CAD build for the part. Positions are in the model's coordinates, mm. A direction names the side the tool comes from. Round coordinates to 2 decimals unless told otherwise and drop trailing zeros. Order: outer loops, then holes, each group sorted by start corner. A loop starts at its lowest first (then second) coordinate and runs counter-clockwise, first axis right, second up. Notation, with made-up numbers: (34.5, 5) -> (83.5, 5) arc R28 ccw to (83.5, 25) -> close; hole circle Ø4 at (43, 5). An arc over 180 degrees is marked (long way). Return JSON: item names as keys, results as strings. Group by question number.
Q1. Cut at B-B (x = -155.5). Write the cut outline in (y, z).
Q2. Mould opens along Z. For faces 1 (the flat face through (185, 13.5, -14)), 2 (the flat face through (14, 13.5, 185)), 3 (the flat face through (161, 32, 37.5)) say: +Z half, -Z half, draft (parallel to the pull), parting line (faces both ways), or undercut.
Q3. Flat gauge pins, fed straight in: pin 1 (3 mm diameter, centred on x = -183.5, z = -15.5, fed in from +Y); pin 2 (8 mm diameter, centred on y = 81.5, z = -47, fed in from -X); pin 3 (1.5 mm diameter, centred on y = 43.5, z = -18.5, fed in from -X). Where does each tip first touch, or does it go through?
Q4. Which spindle directions (+Z, -Z, +X, -X, +Y, -Y) get a long thin tool onto all of the face, cutting with end or side? Do faces 4 (the flat face through (33, 65, 157)), 5 (the flat face through (-120.878, 44.58, -71.982)), 6 (the flat face through (-172, 10, -1)). Say none if no direction does.
Q5. Cut at A-A (x = 0). Write the cut outline in (y, z).
Q6. Probe line 1 along X through (y, z) = (50.5, 162); line 2 along Y through (x, z) = (-61, 22); line 3 along Z through (x, y) = (71, 27.5). List the from-to ranges inside material, lowest first.
from build123d import *

# Parameters (mm, degrees)
SKETCH1_R                    = 150
BOSS_EXTRUDE1_DEPTH          = 75
CHAMFER1_SIZE                = 10
BOSS_EXTRUDE2_START          = -75
BOSS_EXTRUDE2_DEPTH          = 10
CHAMFER2_SIZE                = 10
BOSS_EXTRUDE3_DEPTH          = 10
BOSS_EXTRUDE4_DEPTH          = 3.5
CIRPATTERN1_COUNT            = 4
CIRPATTERN1_COPY_1_DEPTH     = 10
CIRPATTERN1_COPY_2_DEPTH     = 10
CIRPATTERN1_COPY_3_DEPTH     = 10
CIRPATTERN1_COPY_4_DEPTH     = 3.5
CIRPATTERN1_COPY_5_DEPTH     = 3.5
CIRPATTERN1_COPY_6_DEPTH     = 3.5
CHAMFER2_OF_CIRPATTERN1_SIZE = 10
CUT_EXTRUDE1_START           = -60
CUT_EXTRUDE1_DEPTH           = 60
CIRPATTERN3_COUNT            = 4
SKETCH15_R                   = 110
BOSS_EXTRUDE6_DEPTH          = 9
BOSS_EXTRUDE6_TAPER          = 45
SKETCH16_R                   = 15
BOSS_EXTRUDE7_DEPTH          = 20


# Read off the part's stored shape, not the designer's step: Cut-Extrude1
with BuildPart() as part:
    # Sketch1 → Boss-Extrude1 (new body)
    with BuildSketch(Plane(origin=(0, 0, 0), x_dir=(1, 0, 0), z_dir=(0, 1, 0))):
        with Locations(Location((0, 0, 0), (0, 0, 270))):
            Circle(SKETCH1_R)
    extrude(amount=BOSS_EXTRUDE1_DEPTH)

    # Chamfer1
    chamfer1_edges = [part.edges().sort_by_distance(p)[0] for p in [
        (0, 75, -150),
    ]]
    chamfer(chamfer1_edges, length=CHAMFER1_SIZE)

    # Sketch2 → Boss-Extrude2 (add)
    with BuildSketch(Plane(origin=(0, 75, 0), x_dir=(1, 0, 0), z_dir=(0, 1, 0)).offset(BOSS_EXTRUDE2_START)):
        with BuildLine():
            ThreePointArc((-145.236875483, -37.5), (-148.80445444, -18.900643872), (-150, 0))
            Line((-150, 0), (-195.236875483, 0))
            Line((-195.236875483, 0), (-195.236875483, -37.5))
            Line((-195.236875483, -37.5), (-145.236875483, -37.5))
        make_face()
        with BuildLine():
            Line((-195.236875483, 0), (-150, 0))
            ThreePointArc((-150, 0), (-148.80445444, 18.900643872), (-145.236875483, 37.5))
            Line((-145.236875483, 37.5), (-195.236875483, 37.5))
            Line((-195.236875483, 37.5), (-195.236875483, 0))
        make_face()
    boss_extrude2 = extrude(amount=BOSS_EXTRUDE2_DEPTH)

    # Chamfer2
    chamfer2_edges = [part.edges().sort_by_distance(p)[0] for p in [
        (-195.236875483, 5, -37.5),
        (-195.236875483, 5, 37.5),
    ]]
    chamfer(chamfer2_edges, length=CHAMFER2_SIZE)

    # Sketch5 → Boss-Extrude3 (add)
    with BuildSketch(Plane.XY.offset(37.5)):
        Polygon((-145.236875483, 10), (-145.236875483, 65), (-168.236875483, 65), (-185.236875483, 10), align=None)
    boss_extrude3 = extrude(amount=-BOSS_EXTRUDE3_DEPTH)

    # Sketch7 → Boss-Extrude4 (add)
    with BuildSketch(Plane(origin=(0, 10, 0), x_dir=(1, 0, 0), z_dir=(0, 1, 0))):
        Polygon((-180.034917045, -11.010056312), (-185.225263454, -8), (-190.427221891, -10.989943688), (-190.43883392, -16.989943688), (-185.248487512, -20), (-180.046529075, -17.010056312), align=None)
    boss_extrude4 = extrude(amount=BOSS_EXTRUDE4_DEPTH)

    # Mirror2: Boss-Extrude3, Boss-Extrude4 across plane
    add(boss_extrude3.mirror(Plane.XY))
    add(boss_extrude4.mirror(Plane.XY))

    # CirPattern1: Boss-Extrude2, Boss-Extrude3, Boss-Extrude4 ×4 about axis
    cirpattern1_axis = Axis((0, 0, 0), (0, 1, 0))
    add([boss_extrude2.rotate(cirpattern1_axis, i * 360 / CIRPATTERN1_COUNT) for i in range(1, CIRPATTERN1_COUNT)])
    add([boss_extrude3.rotate(cirpattern1_axis, i * 360 / CIRPATTERN1_COUNT) for i in range(1, CIRPATTERN1_COUNT)])
    add([boss_extrude4.rotate(cirpattern1_axis, i * 360 / CIRPATTERN1_COUNT) for i in range(1, CIRPATTERN1_COUNT)])

    # CirPattern1 copy 1 sketch → CirPattern1 copy 1 (add)
    with BuildSketch(Plane(origin=(-37.5, 0, 0), x_dir=(0, 0, -1), z_dir=(-1, 0, 0))):
        Polygon((-145.236875483, -10), (-145.236875483, -65), (-168.236875483, -65), (-185.236875483, -10), align=None)
    extrude(amount=-CIRPATTERN1_COPY_1_DEPTH)

    # CirPattern1 copy 2 sketch → CirPattern1 copy 2 (add)
    with BuildSketch(Plane(origin=(0, 0, 37.5), x_dir=(-1, 0, 0), z_dir=(0, 0, 1))):
        Polygon((-145.236875483, -10), (-145.236875483, -65), (-168.236875483, -65), (-185.236875483, -10), align=None)
    extrude(amount=-CIRPATTERN1_COPY_2_DEPTH)

    # CirPattern1 copy 3 sketch → CirPattern1 copy 3 (add)
    with BuildSketch(Plane(origin=(37.5, 0, 0), x_dir=(0, 0, 1), z_dir=(1, 0, 0))):
        Polygon((-145.236875483, -10), (-145.236875483, -65), (-168.236875483, -65), (-185.236875483, -10), align=None)
    extrude(amount=-CIRPATTERN1_COPY_3_DEPTH)

    # CirPattern1 copy 4 sketch → CirPattern1 copy 4 (add)
    with BuildSketch(Plane(origin=(0, 10, 0), x_dir=(0, 0, -1), z_dir=(0, 1, 0))):
        Polygon((-180.034917045, 11.010056312), (-185.225263454, 8), (-190.427221891, 10.989943688), (-190.43883392, 16.989943688), (-185.248487512, 20), (-180.046529075, 17.010056312), align=None)
    extrude(amount=CIRPATTERN1_COPY_4_DEPTH)

    # CirPattern1 copy 5 sketch → CirPattern1 copy 5 (add)
    with BuildSketch(Plane(origin=(0, 10, 0), x_dir=(-1, 0, 0), z_dir=(0, 1, 0))):
        Polygon((-180.034917045, 11.010056312), (-185.225263454, 8), (-190.427221891, 10.989943688), (-190.43883392, 16.989943688), (-185.248487512, 20), (-180.046529075, 17.010056312), align=None)
    extrude(amount=CIRPATTERN1_COPY_5_DEPTH)

    # CirPattern1 copy 6 sketch → CirPattern1 copy 6 (add)
    with BuildSketch(Plane.ZX.offset(10)):
        Polygon((-180.034917045, 11.010056312), (-185.225263454, 8), (-190.427221891, 10.989943688), (-190.43883392, 16.989943688), (-185.248487512, 20), (-180.046529075, 17.010056312), align=None)
    extrude(amount=CIRPATTERN1_COPY_6_DEPTH)

    # Chamfer2 of CirPattern1
    chamfer2_of_cirpattern1_edges = [part.edges().sort_by_distance(p)[0] for p in [
        (-37.5, 5, 195.236875483),
        (37.5, 5, 195.236875483),
        (195.236875483, 5, 37.5),
        (195.236875483, 5, -37.5),
        (37.5, 5, -195.236875483),
        (-37.5, 5, -195.236875483),
    ]]
    chamfer(chamfer2_of_cirpattern1_edges, length=CHAMFER2_OF_CIRPATTERN1_SIZE)

    # Cut-Extrude1 outline → Cut-Extrude1 (cut)
    with BuildSketch(Plane(origin=(0, 75, 0), x_dir=(1, 0, 0), z_dir=(0, 1, 0)).offset(CUT_EXTRUDE1_START)):
        with BuildLine():
            ThreePointArc((-65, -112.583302492), (-91.923881554, -91.923881554), (-112.583302492, -65))
            Line((-112.583302492, -65), (-129.903810568, -75))
            ThreePointArc((-129.903810568, -75), (-106.066017178, -106.066017178), (-75, -129.903810568))
            Line((-75, -129.903810568), (-65, -112.583302492))
        make_face()
    cut_extrude1 = extrude(amount=CUT_EXTRUDE1_DEPTH, mode=Mode.SUBTRACT)

    # CirPattern3: Cut-Extrude1 ×4 about axis
    cirpattern3_axis = Axis((1.096442134, 0, -1.096442134), (0, 1, 0))
    for i in range(1, CIRPATTERN3_COUNT):
        add(cut_extrude1.rotate(cirpattern3_axis, i * 360 / CIRPATTERN3_COUNT), mode=Mode.SUBTRACT)

    # Sketch15 → Boss-Extrude6 (add)
    with BuildSketch(Plane(origin=(0, 75, 0), x_dir=(1, 0, 0), z_dir=(0, 1, 0))):
        Circle(SKETCH15_R)
    extrude(amount=BOSS_EXTRUDE6_DEPTH, taper=BOSS_EXTRUDE6_TAPER)

    # Sketch16 → Boss-Extrude7 (add)
    with BuildSketch(Plane(origin=(0, 84, 0), x_dir=(1, 0, 0), z_dir=(0, 1, 0))):
        with Locations(Location((0, 0, 0), (0, 0, 270))):
            Circle(SKETCH16_R)
    extrude(amount=BOSS_EXTRUDE7_DEPTH)


solid = part.part
Solution:
{
 "1": {"outline": "(0, -37.5) -> (65, -37.5) -> (65, -27.5) -> (10, -27.5) -> (10, 27.5) -> (65, 27.5) -> (65, 37.5) -> (0, 37.5) -> close"},
 "2": {"face 1": "undercut", "face 2": "draft", "face 3": "+Z half"},
 "3": {"pin 1": "stops at y = 13.5", "pin 2": "stops at x = -97.07", "pin 3": "stops at x = -148.95"},
 "4": {"face 4": "+Z, +X, +Y", "face 5": "-Z, +Y", "face 6": "+Y"},
 "5": {"outline": "(0, -195.24) -> (10, -195.24) -> (10, -150) -> (65, -150) -> (75, -140) -> (75, -110) -> (84, -101) -> (84, -15) -> (104, -15) -> (104, 15) -> (84, 15) -> (84, 101) -> (75, 110) -> (75, 140) -> (65, 150) -> (10, 150) -> (10, 195.24) -> (0, 195.24) -> close"},
 "6": {"line 1": "x = -37.5 to -27.5, 27.5 to 37.5", "line 2": "y = 0 to 84", "line 3": "z = -132.13 to -121.37, -112.49 to 110.3, 119.18 to 132.13"}
}
